Part model, mm, in its own coordinate system. Face numbers are marked on the shaded views. A direction names the side the tool comes from. Round coordinates to 2 decimals unless told otherwise and drop trailing zeros. Loops run counter-clockwise (first coordinate to the right, second up) from the corner with the lowest first, then second, coordinate; pieces in that order, holes last. Notation, with made-up numbers: M -0.5,33 L 41.5,33 A32 ccw 41.5,66 Z; hole C -16.75,-10.5 d5. An arc over 180 degrees is marked long. Put each result on its own line as item: value. Start each with the question number.
1) Slice it at C-C on z = 44.5. Give the cut face in (x, y).
2) Slice it at B-B on x = 44. Give the cut face in (y, z).
3) Probe line 1 along X through (y, z) = (24, 27.5); line 2 along Y through (x, z) = (24, 44); line 3 along Z through (x, y) = (13.5, 47). List the from-to ranges inside material, lowest first.
4) Which spindle directions (+Z, -Z, +X, -X, +Y, -Y) get a long thin tool onto all of the face, cutting with end or side? Do the marked faces 1, 2 and 3. Say none if no direction does.
5) Drop flat-ended pins along their axis: pin 1 Ø10 at (x, z) = (31.5, 33) entering from +Y; pin 2 Ø7.5 at (y, z) = (20, 32.5) entering from +X; pin 3 Ø2 at (x, y) = (23, 38) entering from +Z. Give the stop position or say it passes through.
6) Slice it at D-D on x = 14.5. Give the cut face in (y, z).
7) Slice it at A-A on y = 3. Give the cut face in (x, z).
```python
from build123d import *

# Parameters (mm, degrees)
F0_W      = 50
F0_H      = 50
F1_DEPTH  = 25
F2_W      = 28.057508
F2_H      = 20.635585
F3_DEPTH  = 25
F3_FACE_W = 28.057508
F3_FACE_H = 25
F4_DEPTH  = 13.969657


with BuildPart() as f1:
    # F0 (on Top) → F1 (new body)
    with BuildSketch(Plane.XY):
        with Locations((25, 25)):
            Rectangle(F0_W, F0_H)
    extrude(amount=F1_DEPTH)

    # F2 (on face) → F3 (join)
    with BuildSketch(Plane.XY.offset(25)):
        with Locations((25.881764, 24.287449)):
            Rectangle(F2_W, F2_H)
    extrude(amount=F3_DEPTH)

    # F3_face (on face) → F4 (join, through all)
    with BuildSketch(Plane(origin=(25.881764, 13.969657, 37.5), x_dir=(1, 0, 0), z_dir=(0, -1, 0))):
        Rectangle(F3_FACE_W, F3_FACE_H)
    extrude(amount=F4_DEPTH)


solid = f1.part
```
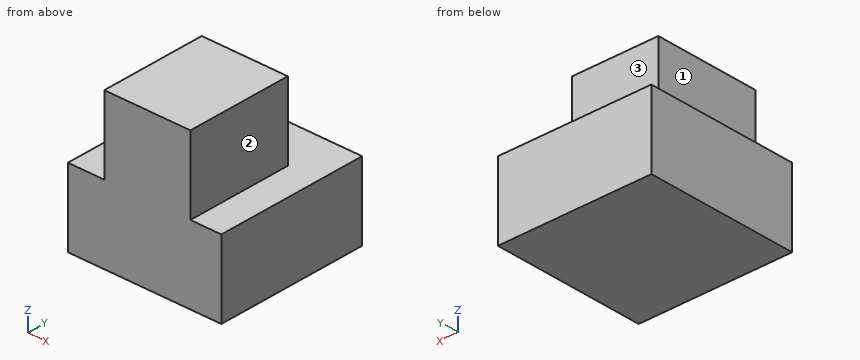
Recorded:
1. outline: M 11.85,0 L 39.91,0 L 39.91,34.61 L 11.85,34.61 Z
2. outline: M 0,0 L 50,0 L 50,25 L 0,25 Z
3. line 1: x = 11.85 to 39.91
3. line 2: y = 0 to 34.61
3. line 3: z = 0 to 25
4. face 1: +Z, -X, +Y, -Y
4. face 2: +Z, +X, +Y, -Y
4. face 3: +Z, +X, -X, +Y
5. pin 1: stops at y = 34.61
5. pin 2: stops at x = 39.91
5. pin 3: stops at z = 25
6. outline: M 0,0 L 50,0 L 50,25 L 34.61,25 L 34.61,50 L 0,50 Z
7. outline: M 0,0 L 50,0 L 50,25 L 39.91,25 L 39.91,50 L 11.85,50 L 11.85,25 L 0,25 Z
